Read the model definition and answer for the solid it produces. Units are mm, in the model's axes. Round coordinates to 2 decimals unless told otherwise and drop trailing zeros. Write each loop counter-clockwise with the first axis right and the second up, starting at its lowest first coordinate (ties: lowest second). Pieces come first, ordered by that corner, then holes. Notation, with made-up numbers: (73.5, 40) - (94.5, 40) arc R19 ccw to (94.5, 49) - close; hole circle Ø9 at (59, -13.5). An arc over 180 degrees is marked (long way). Use one line per item in the form item = value. Start each with the question number.
1) The part is cut by section C-C, the plane z = 2.5. Give the vertices of the cut face in (x, y), plus the area to 3 significant figures.
2) The part is cut by section A-A, the plane y = 0. Give the vertices of the cut face in (x, z), plus the area to 3 significant figures.
3) Consider line 1 along Y through (x, z) = (-45, 2.7); line 2 along X through (y, z) = (8, 0.25); line 3 along X through (y, z) = (-8.5, 4.2). Determine where each line is inside the solid, lowest interval first. Write a range as from..to.
4) For a pull along X with two mould halves and no side action, classify faces 1 (the face through (-55, 0, 2)), 2 (the face through (-1, 0, 5)), 3 (the face through (58.57, 16, 2.54)) as released by +X, released by -X, zero draft, split by the parting line, or undercut.
5) The part is cut by section B-B, the plane x = -45. Give the vertices of the cut face in (y, z).
6) This flat-tipped pin is pushed along its axis until it touches: pin 1 (2 mm diameter, centred on x = -32, y = -10, fed in from -Z). Where does it stop, or does it pass through?
from build123d import *

# Parameters (mm, degrees)
F0_W     = 120
F0_H     = 35
F0_R     = 10
F1_DEPTH = 5
F2_R     = 5
F3_R     = 5


with BuildPart() as f1:
    # F0 (on Top) → F1 (new body)
    with BuildSketch(Plane.XY):
        Rectangle(F0_W, F0_H)
        with Locations((-45, 0)):
            Circle(F0_R, mode=Mode.SUBTRACT)
    extrude(amount=F1_DEPTH)

    # F2
    f2_edges = [f1.edges().sort_by_distance(p)[0] for p in [
        (60, -17.5, 2.5),
    ]]
    fillet(f2_edges, radius=F2_R)

    # F3
    f3_edges = [f1.edges().sort_by_distance(p)[0] for p in [
        (60, 17.5, 2.5),
    ]]
    fillet(f3_edges, radius=F3_R)


solid = f1.part
Geometry results:
q1.outline = (-60, -17.5) - (55, -17.5) arc R5 ccw to (60, -12.5) - (60, 12.5) arc R5 ccw to (55, 17.5) - (-60, 17.5) - close; hole circle Ø20 at (-45, 0)
q1.area = 3,880 mm2
q2.outline = (-60, 0) - (-55, 0) - (-55, 5) - (-60, 5) - close; (-35, 0) - (60, 0) - (60, 5) - (-35, 5) - close
q2.area = 500 mm2
q3.line_1 = -17.5..-10, 10..17.5
q3.line_2 = -60..-51, -39..60
q3.line_3 = -60..-50.27, -39.73..60
q4.face_1 = undercut
q4.face_2 = zero draft
q4.face_3 = released by +X
q5.outline = (-17.5, 0) - (-10, 0) - (-10, 5) - (-17.5, 5) - close; (10, 0) - (17.5, 0) - (17.5, 5) - (10, 5) - close
q6.pin_1 = 0
